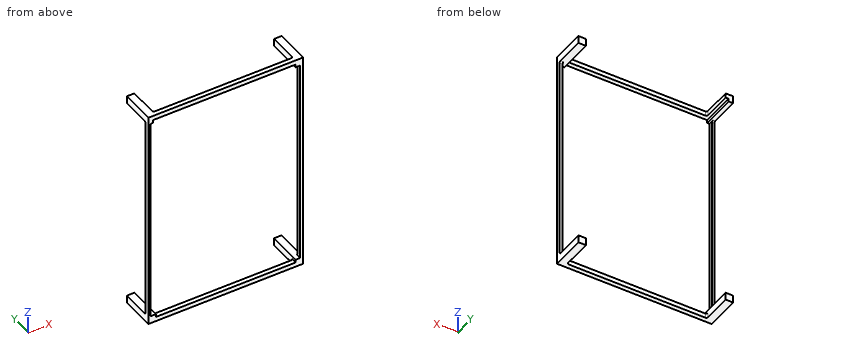
```python
from build123d import *

# Parameters (mm, degrees)
BOSS_EXTRUDE1_DEPTH = 3
SKETCH2_W           = 5
SKETCH2_H           = 5
BOSS_EXTRUDE2_DEPTH = 20
FILLET1_R           = 1


with BuildPart() as part:
    # Sketch1 → Boss-Extrude1 (new body)
    with BuildSketch(Plane(origin=(0, 0, 0), x_dir=(1, 0, 0), z_dir=(0, 1, 0))):
        Polygon((0, 0), (0, 149), (5, 149), (103.25, 149), (103.25, 0), align=None)
        Polygon((98.25, 146), (5, 146), (5, 144), (1.5, 144), (1.5, 5), (3, 5), (3, 3), (5, 3), (98.25, 3), (98.25, 5), (101.25, 5), (101.25, 144), (98.25, 144), align=None, mode=Mode.SUBTRACT)
    extrude(amount=BOSS_EXTRUDE1_DEPTH)

    # Sketch2 → Boss-Extrude2 (add)
    with BuildSketch(Plane(origin=(0, 3, 0), x_dir=(1, 0, 0), z_dir=(0, 1, 0))):
        Polygon((0, 0), (5, 0), (5, 3), (3, 3), (3, 5), (0, 5), align=None)
        with Locations((100.75, 146.5)):
            Rectangle(SKETCH2_W, SKETCH2_H)
        with Locations((2.5, 146.5)):
            Rectangle(SKETCH2_W, SKETCH2_H)
        with Locations((100.75, 2.5)):
            Rectangle(SKETCH2_W, SKETCH2_H)
    extrude(amount=BOSS_EXTRUDE2_DEPTH)

    # Fillet1
    fillet1_edges = [part.edges().sort_by_distance(p)[0] for p in [
        (0.75, 3, -5),
        (102.25, 3, -144),
        (98.25, 3, -147.5),
        (0.75, 3, -144),
        (5, 3, -147.5),
        (98.25, 3, -1.5),
        (102.25, 3, -5),
        (5, 3, -1.5),
    ]]
    fillet(fillet1_edges, radius=FILLET1_R)


solid = part.part
```
Source: CAD feature listing. Evaluate the final solid. Frame: model axes, mm. Round coordinates to 2 decimals unless told otherwise and drop trailing zeros. Loops run counter-clockwise (first coordinate to the right, second up) from the corner with the lowest first, then second, coordinate; pieces in that order, holes last.
1. Ray query, L1, parallel to X at y = 2.75, z = -44.5. Return the intervals inside material, ascending.
2. Section query A-A on x = 24. Output: boundary loops of the cut face in (y, z), and give its area (3 significant figures).
3. Contact query for flat-ended pins moving along their axis: pin 1 (4 mm diameter, centred on x = 100.5, y = 7.5, fed in from +Z); pin 2 (0.6 mm diameter, centred on x = 102.5, z = -93.5, fed in from +Y). Output: stop coordinate, or through.
4. Section query C-C on y = 13. Output: boundary loops of the cut face in (x, z), and give its area (3 significant figures).
5. Section query B-B on z = -136.5. Output: boundary loops of the cut face in (x, y), and give its area (3 significant figures).
Answers below:
1. L1: x = 0 to 1.5, 101.25 to 103.25
2. outline: (0, -149) - (3, -149) - (3, -146) - (0, -146) - close; (0, -3) - (3, -3) - (3, 0) - (0, 0) - close
2. area: 18.0 mm2
3. pin 1: stops at z = 0
3. pin 2: stops at y = 3
4. outline: (0, -149) - (5, -149) - (5, -144) - (0, -144) - close; (0, -5) - (3, -5) - (3, -3) - (5, -3) - (5, 0) - (0, 0) - close; (98.25, -149) - (103.25, -149) - (103.25, -144) - (98.25, -144) - close; (98.25, -5) - (103.25, -5) - (103.25, 0) - (98.25, 0) - close
4. area: 96.0 mm2
5. outline: (0, 0) - (1.5, 0) - (1.5, 3) - (0, 3) - close; (101.25, 0) - (103.25, 0) - (103.25, 3) - (101.25, 3) - close
5. area: 10.5 mm2
